Geometry: see drawing. Coordinates: mm, zero at the bounding-box minimum. Give positions to 0.01 mm unless a question says otherwise; leave off trailing zeros. Loops run counter-clockwise (first coordinate to the right, second up) from the corner with the lowest first, then second, coordinate; pieces in that order, holes last. Notation, with made-up numbers: M -9,-25 L -5,-25 A29 ccw -5,-1 Z; hole C 43,-17.5 d5. An arc over 180 degrees is marked long. Put each result on its own line as item: value.
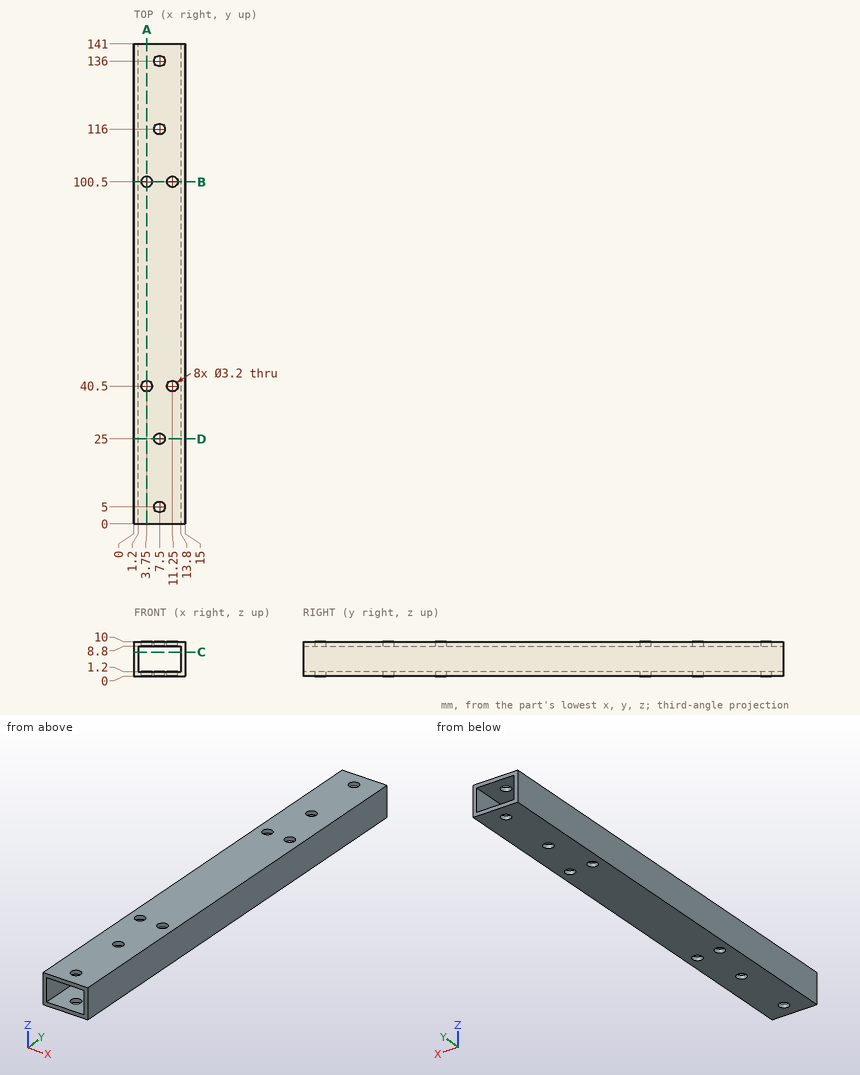
1. Contact query for a flat-ended pin moving along its axis: P1, Ø2.5, axis at x = 3.75, y = 40.5, coming from the +Z side. Output: stop coordinate, or through.
Found:
P1: through
2. Material intervals for line 1 (X direction, y = 100.5, z = 0.4); line 2 (Y direction, x = 7.5, z = 0.5); line 3 (Y direction, x = 3.75, z = 9.2), sorted ascending. Write a range as from..to.
Found:
line 1: 0..2.15, 5.35..9.65, 12.85..15
line 2: 0..3.4, 6.6..23.4, 26.6..114.4, 117.6..134.4, 137.6..141
line 3: 0..38.9, 42.1..98.9, 102.1..141
3. Section query A-A (x = 3.75). Output: boundary loops of the cut face in (y, z), plus the area to 3 significant figures.
Found:
outline: M 0,0 L 38.9,0 L 38.9,1.2 L 0,1.2 Z; M 0,8.8 L 38.9,8.8 L 38.9,10 L 0,10 Z; M 42.1,0 L 98.9,0 L 98.9,1.2 L 42.1,1.2 Z; M 42.1,8.8 L 98.9,8.8 L 98.9,10 L 42.1,10 Z; M 102.1,0 L 141,0 L 141,1.2 L 102.1,1.2 Z; M 102.1,8.8 L 141,8.8 L 141,10 L 102.1,10 Z
area: 323 mm^2
4. Section query D-D (y = 25). Output: boundary loops of the cut face in (x, z), plus the area to 3 significant figures.
Found:
outline: M 0,0 L 5.9,0 L 5.9,1.2 L 1.2,1.2 L 1.2,8.8 L 5.9,8.8 L 5.9,10 L 0,10 Z; M 9.1,0 L 15,0 L 15,10 L 9.1,10 L 9.1,8.8 L 13.8,8.8 L 13.8,1.2 L 9.1,1.2 Z
area: 46.6 mm^2
5. Section query C-C (z = 7). Output: boundary loops of the cut face in (x, y), plus the area to 3 significant figures.
Found:
outline: M 0,0 L 1.2,0 L 1.2,141 L 0,141 Z; M 13.8,0 L 15,0 L 15,141 L 13.8,141 Z
area: 338 mm^2
6. Section query B-B (y = 100.5). Output: boundary loops of the cut face in (x, z), plus the area to 3 significant figures.
Found:
outline: M 0,0 L 2.15,0 L 2.15,1.2 L 1.2,1.2 L 1.2,8.8 L 2.15,8.8 L 2.15,10 L 0,10 Z; M 5.35,0 L 9.65,0 L 9.65,1.2 L 5.35,1.2 Z; M 5.35,8.8 L 9.65,8.8 L 9.65,10 L 5.35,10 Z; M 12.85,0 L 15,0 L 15,10 L 12.85,10 L 12.85,8.8 L 13.8,8.8 L 13.8,1.2 L 12.85,1.2 Z
area: 38.9 mm^2
